Check sheet for the modelled part. Datum: model origin and axes. Units: mm. Give positions to 0.01 mm unless a question says otherwise; leave off trailing zeros. Loops run counter-clockwise (first coordinate to the right, second up) from the corner with the lowest first, then second, coordinate; pieces in that order, holes last.
```python
from build123d import *

# Parameters (mm, degrees)
F1_DEPTH = 9.525
F2_R     = 127


with BuildPart() as f1:
    # F0 (on Front) → F1 (new body)
    with BuildSketch(Plane.XZ):
        with BuildLine():
            ThreePointArc((-609.6, 0), (0, -163.341827706), (609.6, 0))
            ThreePointArc((609.6, 0), (446.258172294, 609.6), (0, 1055.858172294))
            ThreePointArc((0, 1055.858172294), (-446.258172294, 609.6), (-609.6, 0))
        make_face()
    extrude(amount=F1_DEPTH)

    # F2
    f2_edges = [f1.edges().sort_by_distance(p)[0] for p in [
        (0, -4.7625, 1055.858172),
        (-609.6, -4.7625, 0),
        (609.6, -4.7625, 0),
    ]]
    fillet(f2_edges, radius=F2_R)


solid = f1.part
```
(1) Material ranges on line 1 (Z direction, x = -297, y = -2.25); line 2 (Z direction, x = -358.5, y = -1); line 3 (X direction, y = -3, z = -2), recorded low to high.
(2) Section check B-B on x = 306. Record the boundary of the cut face in (y, z) (3 decimals).
(3) Section check A-A on z = 541. Record the boundary of the cut face in (x, y) (3 decimals), plus the area to 3 significant figures.
(4) Gauge pin test, flat ends, axial feed: pin 1 Ø3 at (x, y) = (201, -6) entering from -Z; pin 2 Ø5 at (x, y) = (247, -4.5) entering from -Z; pin 3 Ø1.5 at (y, z) = (-7, 867.5) entering from -X. Record the tip position at first contact, or that the pin passes through.
Computed values:
1. line 1: z = -126.61 to 815.18
1. line 2: z = -109.44 to 741.1
1. line 3: x = -581.18 to 581.18
2. outline: (-9.525, -124.317) - (0, -124.317) - (0, 805.062) - (-9.525, 805.062) - close
3. outline: (-482.997, -9.525) - (482.997, -9.525) - (482.997, 0) - (-482.997, 0) - close
3. area: 9,200 mm2
4. pin 1: stops at z = -146.91
4. pin 2: stops at z = -138.57
4. pin 3: stops at x = -247.83
